Source: CAD feature listing. Evaluate the final solid. Frame: model axes, mm. A direction names the side the tool comes from. Give positions to 0.01 mm unless a question says otherwise; leave off trailing zeros. Loops run counter-clockwise (first coordinate to the right, second up) from the corner with the lowest first, then second, coordinate; pieces in that order, holes last. Notation, with made-up numbers: (-35, 24) -> (-2, 24) arc R7 ccw to (-2, 31) -> close; hole circle Ø7 at (40.25, 21.5). An arc over 180 degrees is marked (long way). Return JSON: item names as keys, results as strings. Group by question number.
```python
from build123d import *

# Parameters (mm, degrees)
SKETCH_W        = 14
SKETCH_H        = 2
PAD_DEPTH       = 3
SKETCH001_W     = 22
SKETCH001_H     = 70
POCKET_DEPTH    = 2
POCKET001_DEPTH = 2
POCKET002_DEPTH = 3.001
CHAMFER_SIZE    = 1.99
CHAMFER001_SIZE = 1.99
FILLET_R        = 2.99


with BuildPart() as part:
    # Sketch → Pad (new body, symmetric)
    with BuildSketch(Plane.XZ):
        Polygon((-26, 0), (-26, 3), (-11, 3), (-11, 70), (11, 70), (11, 3), (26, 3), (26, 0), align=None)
        with Locations((0, 6)):
            Rectangle(SKETCH_W, SKETCH_H, mode=Mode.SUBTRACT)
    extrude(amount=PAD_DEPTH, both=True)

    # Sketch001 (on Face14 of Pad) → Pocket (cut)
    with BuildSketch(Plane.XZ.offset(3)):
        with Locations((0, 38)):
            Rectangle(SKETCH001_W, SKETCH001_H)
    extrude(amount=-POCKET_DEPTH, mode=Mode.SUBTRACT)

    # Sketch002 (on Face16 of Pocket) → Pocket001 (cut)
    with BuildSketch(Plane.XZ.offset(1)):
        Polygon((-9.25, 68), (9.25, 68), (9.25, 13), (7, 13), (7, 7), (-7, 7), (-7, 13), (-9.25, 13), align=None)
    extrude(amount=-POCKET001_DEPTH, mode=Mode.SUBTRACT)

    # Sketch003 (on Face3 of Pocket001) → Pocket002 (cut, through all)
    with BuildSketch(Plane(origin=(0, 0, 3), x_dir=(-1, 0, 0), z_dir=(0, 0, 1))):
        with BuildLine():
            ThreePointArc((-19.59, -1.65), (-17.94, 0), (-19.59, 1.65))
            Line((-19.59, 1.65), (-21.59, 1.65))
            ThreePointArc((-21.59, 1.65), (-23.24, 0), (-21.59, -1.65))
            Line((-19.59, -1.65), (-21.59, -1.65))
        make_face()
        with BuildLine():
            ThreePointArc((19.59, 1.65), (17.94, 0), (19.59, -1.65))
            Line((19.59, -1.65), (21.59, -1.65))
            ThreePointArc((21.59, -1.65), (23.24, 0), (21.59, 1.65))
            Line((19.59, 1.65), (21.59, 1.65))
        make_face()
    extrude(amount=-POCKET002_DEPTH, mode=Mode.SUBTRACT)

    # Chamfer
    chamfer_edges = [part.edges().sort_by_distance(p)[0] for p in [
        (0, -1, 3),
    ]]
    chamfer(chamfer_edges, length=CHAMFER_SIZE)

    # Chamfer001
    chamfer001_edges = [part.edges().sort_by_distance(p)[0] for p in [
        (-11, 1, 3),
        (11, 1, 3),
    ]]
    chamfer(chamfer001_edges, length=CHAMFER001_SIZE)

    # Fillet
    fillet_edges = [part.edges().sort_by_distance(p)[0] for p in [
        (-26, 3, 1.5),
        (-26, -3, 1.5),
        (26, -3, 1.5),
        (26, 3, 1.5),
    ]]
    fillet(fillet_edges, radius=FILLET_R)


solid = part.part
```
1) Contact query for flat-ended pins moving along their axis: P1, Ø6.5, axis at x = 0.5, z = 32, coming from the -Y side; P2, Ø2, axis at y = 1, z = 53, coming from the -X side; P3, Ø20.5, axis at x = -0.5, z = 35.5, coming from the -Y side. Output: stop coordinate, or through.
2) Cut plane C-C on x = -17. Return loops of the section in (y, z), then the cut area to 3 significant figures.
3) Cut plane B-B on z = 21. Return loops of the section in (x, y).
4) Mould query, pull axis X, two halves, no side actions, for faces 5 (the face through (-25.15, 2.1, 1.52)), 6 (the face through (0, 1, 5)), 7 (the face through (-23.24, 0.04, 1.52)), 8 (the face through (-10, -1, 40)). Classes: released by +X, released by -X, zero draft, split by the parting line, or undercut.
5) Reachability of faces 1 (the face through (8, 0, 13)), 2 (the face through (0, 2, 7)), 3 (the face through (11.98, 0.71, 4.01)), 4 (the face through (21, -1.65, 2)) from +Z, -Z, +X, -X, +Y, -Y: full face, straight path, thin tool, end or side. Return the list, or none.
6) Material intervals for line 1 (X direction, y = 0.25, z = 45); line 2 (Z direction, x = 4, y = -0.75); line 3 (Y direction, x = -9.5, z = 49), sorted ascending.
Calculated:
{
 "1": {"P1": "y = 1", "P2": "x = -11", "P3": "y = -1"},
 "2": {"outline": "(-3, 0) -> (3, 0) -> (3, 3) -> (-3, 3) -> close", "area": "18.0 mm2"},
 "3": {"outline": "(-11, -1) -> (-9.25, -1) -> (-9.25, 1) -> (9.25, 1) -> (9.25, -1) -> (11, -1) -> (11, 3) -> (-11, 3) -> close"},
 "4": {"face 5": "released by -X", "face 6": "undercut", "face 7": "undercut", "face 8": "zero draft"},
 "5": {"face 1": "-Y", "face 2": "+Y, -Y", "face 3": "+Z, +X, +Y, -Y", "face 4": "+Z, -Z"},
 "6": {"line 1": "-11 to -9.25, 9.25 to 11", "line 2": "0 to 5, 68 to 70", "line 3": "-1 to 3"}
}
